Geometry check sheet. Reference: the model listing, model coordinates, mm. A direction names the side the tool comes from. Give positions to 0.01 mm unless a question says otherwise; leave off trailing zeros. Write each loop counter-clockwise with the first axis right and the second up, starting at its lowest first coordinate (ties: lowest second). Pieces come first, ordered by that corner, then holes. Notation, with made-up numbers: (-19, 45.5) - (-14, 45.5) arc R28 ccw to (-14, 84.5) - close; hole circle Ø9 at (-9, 20). An arc over 180 degrees is marked (long way). Write item = value, one per line. Start each with the question number.
(1) Section check C-C, the plane z = 10. Enter the section's corners in (x, y) (3 decimals), plus the area to 3 significant figures.
(2) Section check B-B, the plane z = -17. Give the number of separate pieces and of enclosed holes in the cut face, plus the area to 3 significant figures.
(3) Depth check by flat-ended pin: pin 1 Ø20 at (x, z) = (0, 17.5) entering from -Y; pin 2 Ø6.5 at (y, z) = (0, 25.25) entering from -X; pin 3 Ø8 at (y, z) = (-2, -5) entering from -X (3 decimals); pin 4 Ø3 at (y, z) = (0.5, 13.5) entering from +X (3 decimals). Enter the tip coordinate at first touch or a pass-through.
(4) Thickness scan on L1, parallel to Z at x = -22.5, y = 0 (3 decimals); L2, parallel to Z at x = -54, y = 11.5; L3, parallel to X at y = -3, z = -18.5. Record the ranges inside material, lowest first.
(5) Draft check along Y on faces 4 (the cylindrical face through (-56.46, -3.23, -12.32)), 5 (the flat face through (-15, 0, 28)), 6 (the flat face through (-1, -5, 4)), 7 (the cylindrical face through (21.81, 1.15, 23.03)). Enter one of: pulls with the +Y half, pulls with the -Y half, needs draft (parallel to the pull), parting line crosses it, or undercut.
(6) Access from +Z, -Z, +X, -X, +Y, -Y to the whole of each face (thin tool, end or side, straight path). Record for faces 1 (the flat face through (30.625, 0, 15)), 2 (the flat face through (12.75, 0, 28)), 3 (the flat face through (-1, 5, 4)).
```python
from build123d import *

# Parameters (mm, degrees)
F0_R          = 5.3062476442
F0_R_2        = 5.6471789454
F2_DEPTH      = 25
F3_DEPTH      = 5
F3_DEPTH_BACK = 5
F5_D          = 5
F6_R          = 4.99999


# Not quite as in the source:
# - a fillet or chamfer is up to 0.001 mm smaller than in the source, because OpenCascade refuses the exact size


with BuildPart() as f2:
    # F0 (on Top) → F2 (new body)
    with BuildSketch(Plane.XY):
        with BuildLine():
            Line((55.3750023246, 13.3750010282), (-52.2500015795, 13.3750010282))
            ThreePointArc((-52.2500015795, 13.3750010282), (-66.8750023469, -1.2499997392), (-52.2500015795, -15.8750005066))
            Line((-52.2500015795, -15.8750005066), (55.3750023246, -15.8750005066))
            ThreePointArc((55.3750023246, -15.8750005066), (70.000003092, -1.2499997392), (55.3750023246, 13.3750010282))
        make_face()
        with Locations((-52.2500015795, 0)):
            Circle(F0_R, mode=Mode.SUBTRACT)
        with Locations((55.3750023246, 0)):
            Circle(F0_R_2, mode=Mode.SUBTRACT)
    extrude(amount=-F2_DEPTH)

    # F1 (on Front) → F3 (join, two sides)
    with BuildSketch(Plane.XZ) as f3_sk:
        with BuildLine():
            Line((-32.5000025332, 21.8750014901), (-32.5000025332, 0))
            Line((-32.5000025332, 0), (30.625000596, 0))
            Line((30.625000596, 0), (30.625000596, 21.8750014901))
            Line((30.625000596, 21.8750014901), (30.625000596, 30.1250014454))
            Line((30.625000596, 30.1250014454), (12.7500016242, 30.1250014454))
            Line((12.7500016242, 30.1250014454), (12.7500016242, 21.8750014901))
            ThreePointArc((12.7500016242, 21.8750014901), (-1.1874996126, 4.9502638014), (-15.1250008494, 21.8750014901))
            Line((-15.1250008494, 21.8750014901), (-15.000000596, 21.8750014901))
            Line((-15.000000596, 21.8750014901), (-15.000000596, 30.1250014454))
            Line((-15.000000596, 30.1250014454), (-32.5000025332, 30.1250014454))
            Line((-32.5000025332, 30.1250014454), (-32.5000025332, 21.8750014901))
        make_face()
    extrude(amount=F3_DEPTH)
    extrude(f3_sk.sketch, amount=-F3_DEPTH_BACK)

    # F5 (through all)
    with Locations(Plane(origin=(-32.5000025332, 0, 0), x_dir=(0, -1, 0), z_dir=(-1, 0, 0))):
        with Locations((0, 25.2500027418)):
            Hole(F5_D / 2)

    # F6 (radius 5 in the source; OpenCascade refuses exactly that, so slightly less here)
    f6_edges = [f2.edges().sort_by_distance(p)[0] for p in [
        (21.687501, 5, 30.125001),
        (21.687501, -5, 30.125001),
        (-23.750002, 5, 30.125001),
        (-23.750002, -5, 30.125001),
    ]]
    fillet(f6_edges, radius=F6_R)


solid = f2.part
```
Model answer:
q1.outline = (-32.5, -5) - (-12.047, -5) - (-12.047, 5) - (-32.5, 5) - close; (9.672, -5) - (30.625, -5) - (30.625, 5) - (9.672, 5) - close
q1.area = 414 mm²
q2.separate_pieces = 1
q2.enclosed_holes = 2
q2.area = 3,630 mm²
q3.pin_1 = through
q3.pin_2 = -32.5
q3.pin_3 = -66.875
q3.pin_4 = 30.625
q4.L1 = -25 to 22.75, 27.75 to 30.125
q4.L2 = -25 to 0
q4.L3 = -66.77 to -56.63, -47.87 to 50.59, 60.16 to 69.89
q5.face_4 = undercut
q5.face_5 = needs draft
q5.face_6 = pulls with the -Y half
q5.face_7 = undercut
q6.face_1 = +Z, +X, +Y, -Y
q6.face_2 = +Z, +Y, -Y
q6.face_3 = +Z, +X, -X, +Y
